Check sheet for the drawn part. Datum: minimum x, y, z corner. Units: mm. Round coordinates to 2 decimals unless told otherwise and drop trailing zeros. Write each loop counter-clockwise with the first axis right and the second up, starting at its lowest first coordinate (ties: lowest second). Pieces come first, ordered by that corner, then holes. Notation, with made-up numbers: (29.5, 51.25) -> (80.5, 51.25) arc R22 cw to (80.5, 81.25) -> close; hole circle Ø11 at (79, 84). An arc over 180 degrees is marked (long way). One line per item, written item: value. Start each with the question number.
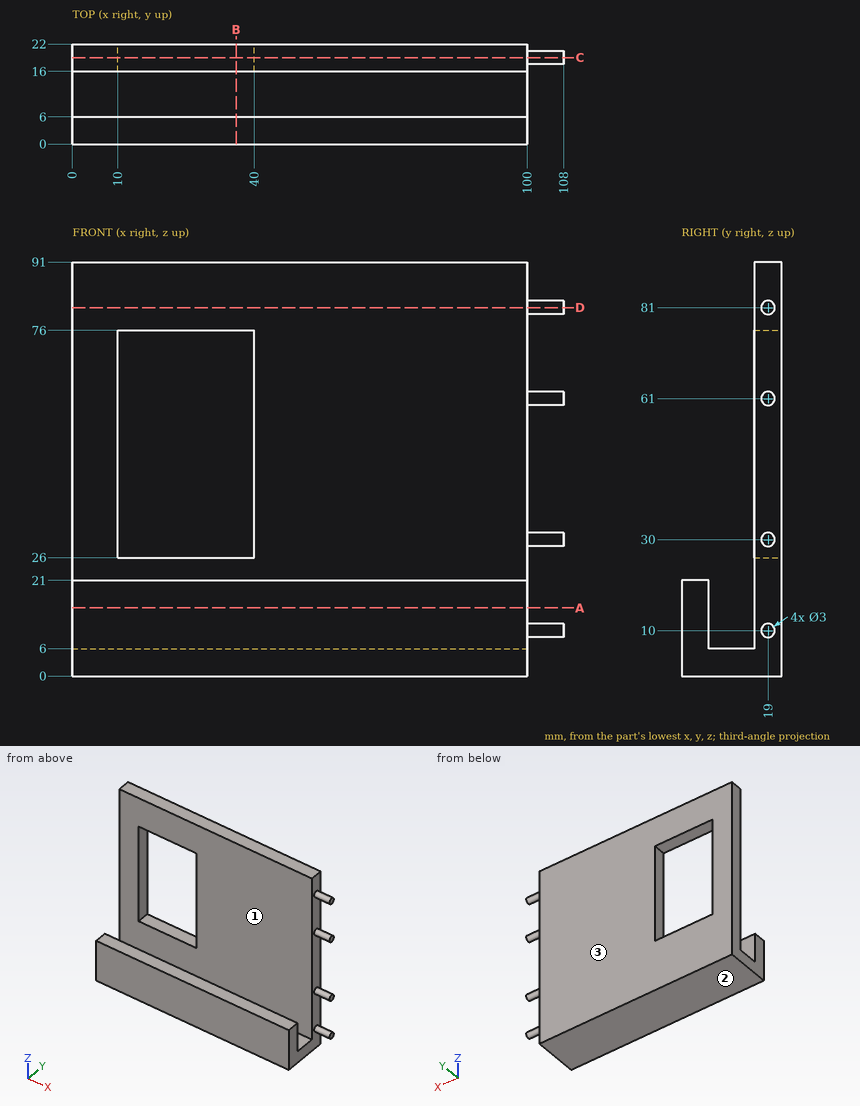
1. Cross-section at B-B (x = 36). Record the cut outline in (y, z).
2. Cross-section at C-C (y = 19). Record the cut outline in (x, z), plus the area to 3 significant figures.
3. Depth check by flat-ended pin: pin 1 Ø1.8 at (x, y) = (36.5, 1.5) entering from +Z; pin 2 Ø3 at (y, z) = (18.5, 55.5) entering from +X; pin 3 Ø3 at (x, y) = (61, 8.5) entering from +Z. Enter the tip coordinate at first touch or a pass-through.
4. Cross-section at D-D (z = 81). Record the cut outline in (x, y).
5. Cross-section at A-A (z = 15). Record the cut outline in (x, y), plus the area to 3 significant figures.
6. Material ranges on probe 1 along Y at (x, z) = (43, 16); probe 2 along Z at (x, y) = (32, 19); probe 3 along X at (y, z) = (18, 59.5), recorded low to high.
7. Release check for a two-part mould opening along Y. For the marked faces 1, 2 and 3 record: +Y half, -Y half, draft (parallel to the pull), parting line (faces both ways), or undercut.
Working result:
1. outline: (0, 0) -> (22, 0) -> (22, 26) -> (16, 26) -> (16, 6) -> (6, 6) -> (6, 21) -> (0, 21) -> close; (16, 76) -> (22, 76) -> (22, 91) -> (16, 91) -> close
2. outline: (0, 0) -> (100, 0) -> (100, 8.5) -> (108, 8.5) -> (108, 11.5) -> (100, 11.5) -> (100, 28.5) -> (108, 28.5) -> (108, 31.5) -> (100, 31.5) -> (100, 59.5) -> (108, 59.5) -> (108, 62.5) -> (100, 62.5) -> (100, 79.5) -> (108, 79.5) -> (108, 82.5) -> (100, 82.5) -> (100, 91) -> (0, 91) -> close; hole (10, 26) -> (40, 26) -> (40, 76) -> (10, 76) -> close
2. area: 7,700 mm^2
3. pin 1: stops at z = 21
3. pin 2: stops at x = 100
3. pin 3: stops at z = 6
4. outline: (0, 16) -> (100, 16) -> (100, 17.5) -> (108, 17.5) -> (108, 20.5) -> (100, 20.5) -> (100, 22) -> (0, 22) -> close
5. outline: (0, 0) -> (100, 0) -> (100, 6) -> (0, 6) -> close; (0, 16) -> (100, 16) -> (100, 22) -> (0, 22) -> close
5. area: 1,200 mm^2
6. probe 1: y = 0 to 6, 16 to 22
6. probe 2: z = 0 to 26, 76 to 91
6. probe 3: x = 0 to 10, 40 to 100
7. face 1: undercut
7. face 2: draft
7. face 3: +Y half
